from build123d import *

# Parameters (mm, degrees)
SKETCH_1_W      = 99.16
SKETCH_1_H      = 115
SKETCH_1_R      = 1.585
SKETCH_1_R_2    = 1.05
SKETCH_1_W_2    = 68
SKETCH_1_H_2    = 106
EXTRUDE_1_DEPTH = 2


with BuildPart() as part:
    # 草图1 → 凸台-拉伸1 (new body)
    with BuildSketch(Plane(origin=(0, 0, 0), x_dir=(1, 0, 0), z_dir=(0, 1, 0))):
        with Locations((49.58, -57.5)):
            Rectangle(SKETCH_1_W, SKETCH_1_H)
        with Locations(Location((90.66, -13.2, 0), (0, 0, 270))):
            Circle(SKETCH_1_R, mode=Mode.SUBTRACT)
        with Locations(Location((90.66, -101.2, 0), (0, 0, 270))):
            Circle(SKETCH_1_R, mode=Mode.SUBTRACT)
        with Locations(Location((8.12, -12.2, 0), (0, 0, 270))):
            Circle(SKETCH_1_R, mode=Mode.SUBTRACT)
        with Locations(Location((8.62, -38.06, 0), (0, 0, 270))):
            Circle(SKETCH_1_R, mode=Mode.SUBTRACT)
        with Locations(Location((15.69, -2, 0), (0, 0, 270))):
            Circle(SKETCH_1_R_2, mode=Mode.SUBTRACT)
        with Locations(Location((78.69, -2, 0), (0, 0, 270))):
            Circle(SKETCH_1_R_2, mode=Mode.SUBTRACT)
        with Locations(Location((15.69, -113, 0), (0, 0, 270))):
            Circle(SKETCH_1_R_2, mode=Mode.SUBTRACT)
        with Locations(Location((78.69, -113, 0), (0, 0, 270))):
            Circle(SKETCH_1_R_2, mode=Mode.SUBTRACT)
        with Locations((47.19, -57.5)):
            Rectangle(SKETCH_1_W_2, SKETCH_1_H_2, mode=Mode.SUBTRACT)
    extrude(amount=EXTRUDE_1_DEPTH)


solid = part.part
Design review of the part built by this model. Coordinates are the model's own, in mm. Give positions to 0.01 mm unless a question says otherwise; leave off trailing zeros. Order: outer loops, then holes, each group sorted by start corner. A loop starts at its lowest first (then second) coordinate and runs counter-clockwise, first axis right, second up. Notation, with made-up numbers: (81, -5.5) - (140, -5.5) arc R12 ccw to (140, 10.5) - close; hole circle Ø11 at (65.25, 88). An arc over 180 degrees is marked (long way). Write item = value, one per line. Start each with the question number.
Q1. We need section B-B on z = 101.2. State the section outline as (x, y) points (3 decimals), plus the area to 3 significant figures.
Q2. To check wall thickness, follow L1, parallel to Z at x = 78.69, y = 0.8; L2, parallel to X at y = 1.25, z = 113; L3, parallel to X at y = 0.9, z = 38.06 (3 decimals). State the ranges of each line that lie inside material, in increasing order. Write a range as from..to.
Q3. We need section C-C on y = 0.6. State how many separate pieces and enclosed holes the cut face has, plus the area to 3 significant figures.
Q4. We need section A-A on x = 90.66. State the section outline as (y, z) points (3 decimals).
Q5. Clearance check with flat-ended pins moving along their axes: pin 1 Ø2.5 at (x, z) = (90.66, 101.2) entering from +Y; pin 2 Ø1 at (x, y) = (86, 1) entering from -Z. State where each tip first meets the part, or that it passes through.
Q6. Mouldability with a two-part tool opening along Z and no side actions: class faces 1 (the face through (92, 0.99, 14.05)), 2 (the face through (82, 0, 57)) as released by +Z, released by -Z, zero draft, split by the parting line, or undercut.
Q7. We need section D-D on x = 35. State the section outline as (y, z) points, plus the area to 3 significant figures.
Working result:
q1.outline = (0, 0) - (13.19, 0) - (13.19, 2) - (0, 2) - close; (81.19, 0) - (89.075, 0) - (89.075, 2) - (81.19, 2) - close; (92.245, 0) - (99.16, 0) - (99.16, 2) - (92.245, 2) - close
q1.area = 56.0 mm²
q2.L1 = 0..0.95, 3.05..4.5, 110.5..111.95, 114.05..115
q2.L2 = 0..14.64, 16.74..77.64, 79.74..99.16
q2.L3 = 0..7.035, 10.205..13.19, 81.19..99.16
q3.separate_pieces = 1
q3.enclosed_holes = 9
q3.area = 4,150 mm²
q4.outline = (0, 0) - (2, 0) - (2, 11.615) - (0, 11.615) - close; (0, 14.785) - (2, 14.785) - (2, 99.615) - (0, 99.615) - close; (0, 102.785) - (2, 102.785) - (2, 115) - (0, 115) - close
q5.pin_1 = through
q5.pin_2 = 0
q6.face_1 = undercut
q6.face_2 = zero draft
q7.outline = (0, 0) - (2, 0) - (2, 4.5) - (0, 4.5) - close; (0, 110.5) - (2, 110.5) - (2, 115) - (0, 115) - close
q7.area = 18.0 mm²
